Could you check a few things on this model? Use its own coordinates, in mm. A direction names the side the tool comes from. Round coordinates to 2 decimals unless told otherwise and drop trailing zeros. Loops run counter-clockwise (first coordinate to the right, second up) from the corner with the lowest first, then second, coordinate; pieces in that order, holes last. Notation, with made-up numbers: (-17.5, 64.25) -> (-11.5, 64.25) arc R31 cw to (-11.5, 90.25) -> close; hole circle Ø2 at (-3.5, 74.5). An arc over 180 degrees is marked (long way). Write each question's results on one line, items separated by ' | '. Start each with the question number.
1) We'd pull the mould along Z, two halves only. Please class faces 5 (the flat face through (0, 40, -10)), 6 (the flat face through (0, 2, 15)), 7 (the flat face through (17.8, 13, -1)): pulls with the +Z half, pulls with the -Z half, needs draft (parallel to the pull), parting line crosses it, or undercut.
2) If I drill on probe 1 along X at (y, z) = (2.5, 0); probe 2 along X at (y, z) = (20, 0); probe 3 along Z at (x, y) = (-20, 27.75), over which ranges is the centre line in solid material (lowest first)?
3) Imagine slicing it at B-B, the plane z = 0. List the corners of the cut face in (x, y) for me, plus the area to 3 significant figures.
4) Imagine slicing it at D-D, the plane y = 11.5. List the corners of the cut face in (x, z) for me, plus the area to 3 significant figures.
5) For P1, Ø4, axis at x = -20, z = 0, coming from the +Y side; P2, Ø6, axis at x = 18, z = -10, coming from the -Y side; P3, Ø9, axis at x = 11, z = -7.5, coming from the -Y side; P4, Ø12, axis at x = -17.5, y = 25.5, coming from the +Z side, each with a flat end and sliding along its axis, tell me the tip position at first contact or that it passes through.
6) Which directions (+Z, -Z, +X, -X, +Y, -Y) give clear straight access to the entire face, cutting with the end or side of a thin tool? Please do faces 1 (the flat face through (0, 0, 10)), 2 (the cylindrical face through (-22.196, 5.902, 0.488)), 3 (the flat face through (0, 0, -9)), 4 (the flat face through (-22.2, 13, -1)).
7) Imagine slicing it at C-C, the plane x = 1.5. List the corners of the cut face in (y, z) for me.
8) Imagine slicing it at A-A, the plane x = 18.5. List the corners of the cut face in (y, z) for me, plus the area to 3 significant figures.
from build123d import *

# Parameters (mm, degrees)
BOSS_EXTRUDE1_DEPTH = 30
SKETCH2_R           = 2.25
CUT_EXTRUDE1_DEPTH  = 53.201532545
CUT_EXTRUDE2_START  = -13
SKETCH3_R           = 5
CUT_EXTRUDE2_DEPTH  = 40.201532545
BOSS_EXTRUDE2_START = 1
SKETCH4_W           = 60
SKETCH4_H           = 8
SKETCH4_R           = 2.25
BOSS_EXTRUDE2_DEPTH = 1


with BuildPart() as part:
    # Sketch1 → Boss-Extrude1 (new, symmetric)
    with BuildSketch(Plane(origin=(0, 0, 0), x_dir=(0, 0, -1), z_dir=(1, 0, 0))):
        Polygon((-15, 0), (15, 0), (15, 40), (5.784609691, 40), (-15, 4), align=None)
    extrude(amount=BOSS_EXTRUDE1_DEPTH, both=True)

    # Sketch2 → Cut-Extrude1 (cut, through all)
    with BuildSketch(Plane.XZ):
        with Locations(Location((-20, 0, 0), (0, 0, 270))):
            Circle(SKETCH2_R)
        with Locations(Location((20, 0, 0), (0, 0, 270))):
            Circle(SKETCH2_R)
    extrude(amount=-CUT_EXTRUDE1_DEPTH, mode=Mode.SUBTRACT)

    # Sketch3 → Cut-Extrude2 (cut, through all)
    with BuildSketch(Plane.XZ.offset(CUT_EXTRUDE2_START)):
        with Locations(Location((-20, 0, 0), (0, 0, 270))):
            Circle(SKETCH3_R)
        with Locations(Location((20, 0, 0), (0, 0, 270))):
            Circle(SKETCH3_R)
    extrude(amount=-CUT_EXTRUDE2_DEPTH, mode=Mode.SUBTRACT)

    # Sketch4 → Boss-Extrude2 (add)
    with BuildSketch(Plane.XZ.offset(BOSS_EXTRUDE2_START)):
        Rectangle(SKETCH4_W, SKETCH4_H)
        with Locations(Location((-20, 0, 0), (0, 0, 270))):
            Circle(SKETCH4_R, mode=Mode.SUBTRACT)
        with Locations(Location((20, 0, 0), (0, 0, 270))):
            Circle(SKETCH4_R, mode=Mode.SUBTRACT)
    extrude(amount=-BOSS_EXTRUDE2_DEPTH)


solid = part.part
Checked values:
1) face 5: needs draft | face 6: pulls with the +Z half | face 7: undercut
2) probe 1: -30 to -22.25, -17.75 to 17.75, 22.25 to 30 | probe 2: -30 to -25, -15 to 15, 25 to 30 | probe 3: -15 to -5
3) outline: (-30, -1) -> (-22.25, -1) -> (-22.25, 13) -> (-25, 13) -> (-25, 29.98) -> (-30, 29.98) -> close; (-17.75, -1) -> (17.75, -1) -> (17.75, 13) -> (15, 13) -> (15, 29.98) -> (-15, 29.98) -> (-15, 13) -> (-17.75, 13) -> close; (22.25, -1) -> (30, -1) -> (30, 29.98) -> (25, 29.98) -> (25, 13) -> (22.25, 13) -> close | area: 1,390 mm^2
4) outline: (-30, -15) -> (30, -15) -> (30, 10.67) -> (-30, 10.67) -> close; hole circle Ø4.5 at (-20, 0); hole circle Ø4.5 at (20, 0) | area: 1,510 mm^2
5) P1: through | P2: y = 0 | P3: y = -1 | P4: z = 6.05
6) face 1: +Z, +X, -X, -Y | face 2: +Y, -Y | face 3: -Z, +X, -X, -Y | face 4: +Y
7) outline: (-1, -4) -> (0, -4) -> (0, -15) -> (40, -15) -> (40, -5.78) -> (4, 15) -> (0, 15) -> (0, 4) -> (-1, 4) -> close
8) outline: (-1, -4) -> (0, -4) -> (0, -15) -> (40, -15) -> (40, -5.78) -> (38.24, -4.77) -> (13, -4.77) -> (13, -1.68) -> (-1, -1.68) -> close; (-1, 1.68) -> (13, 1.68) -> (13, 4.77) -> (21.72, 4.77) -> (4, 15) -> (0, 15) -> (0, 4) -> (-1, 4) -> close | area: 625 mm^2
